The drawing under review shows one solid part. Ordinate dimensions are in mm from its lowest x, y, z. A direction names the side the tool comes from. Coordinates: 2 decimals unless noted, no trailing zeros. Order: outer loops, then holes, each group sorted by start corner. A loop starts at its lowest first (then second) coordinate and runs counter-clockwise, first axis right, second up. Notation, with made-up numbers: (-29, -24.75) - (19, -24.75) arc R7 ccw to (19, -17.75) - close; hole circle Ø4 at (67.5, -38). An arc over 180 degrees is marked (long way). Write item = value, one per line. Start each with the question number.
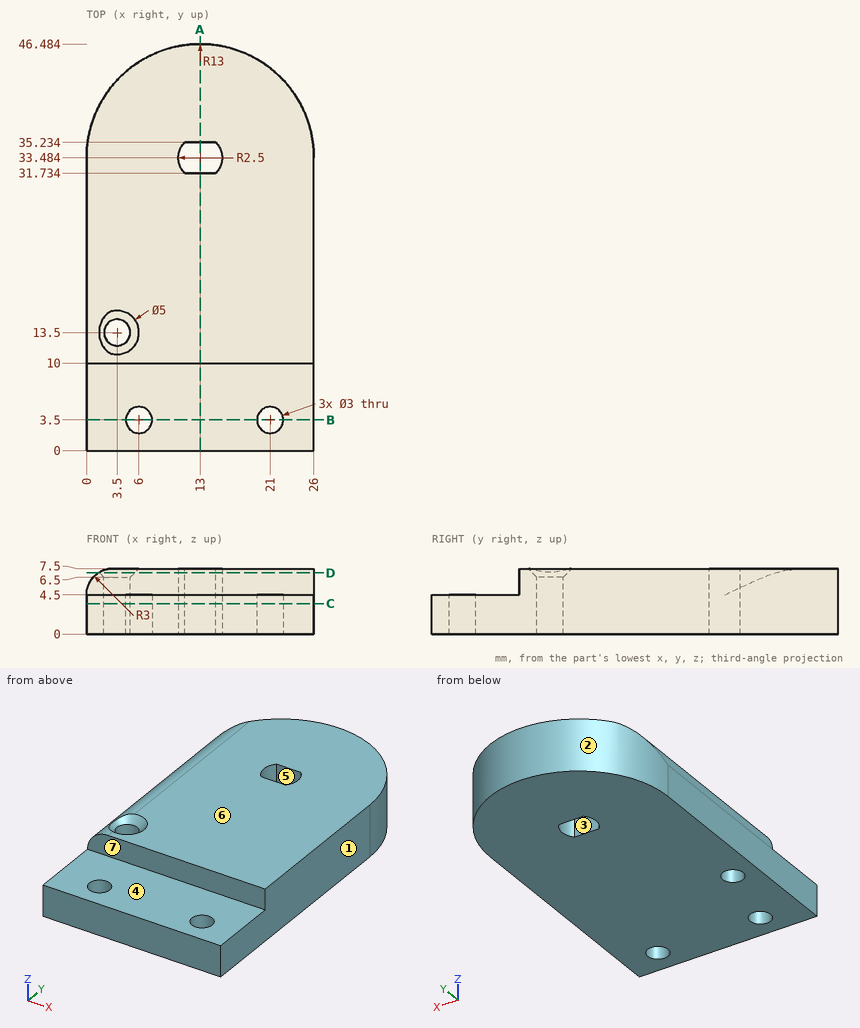
Item 1: For line 1 (X direction, y = 13.5, z = 4); line 2 (Y direction, x = 3.5, z = 2.25); line 3 (Y direction, x = 4, z = 5.75), list the stretches that pass through material, from the lowest coordinate up.
Item 2: For the marked faces 5, 6 and 7, list the 3-axis set-ups (+Z, -Z, +X, -X, +Y, -Y) from which the entire face can be reached by the end or side of a thin tool; tool diameter is ignored.
Item 3: Mouldability with a two-part tool opening along X and no side actions: class the marked faces 1, 2, 3 and 4 as +X half, -X half, draft (parallel to the pull), parting line (faces both ways), or undercut.
Item 4: For P1, Ø5, axis at x = 6, y = 3.5, coming from the +Z side; P2, Ø1.5, axis at x = 15.5, z = 6.5, coming from the -Y side; P3, Ø3, axis at y = 40.5, z = 4, coming from the -X side; P4, Ø1.8, axis at x = 21, y = 3.5, coming from the -Z side, all flat-tipped, find the tip position at first contact; note any pin that passes through.
Item 5: Add section A-A on x = 13. Give the boundary of the cut face in (y, z).
Item 6: Add section B-B on y = 3.5. Give the boundary of the cut face in (x, z), plus the area to 3 significant figures.
Item 7: Add section D-D on z = 7. Give the boundary of the cut face in (x, y), plus the area to 3 significant figures.
Item 8: Add section C-C on z = 3.5. Give the boundary of the cut face in (x, y), plus the area to 3 significant figures.
Worked out:
q1.line_1 = 0 to 2, 5 to 26
q1.line_2 = 0 to 12, 15 to 42.36
q1.line_3 = 10 to 12.09, 14.91 to 42.86
q2.face_5 = +Z, -Z
q2.face_6 = +Z, +X, -X, +Y, -Y
q2.face_7 = +Z, +X, -X, -Y
q3.face_1 = +X half
q3.face_2 = parting line
q3.face_3 = undercut
q3.face_4 = draft
q4.P1 = 4.5
q4.P2 = 10
q4.P3 = 1.23
q4.P4 = through
q5.outline = (0, 0) - (31.73, 0) - (31.73, 7.5) - (10, 7.5) - (10, 4.5) - (0, 4.5) - close; (35.23, 0) - (46.48, 0) - (46.48, 7.5) - (35.23, 7.5) - close
q6.outline = (0, 0) - (4.5, 0) - (4.5, 4.5) - (0, 4.5) - close; (7.5, 0) - (19.5, 0) - (19.5, 4.5) - (7.5, 4.5) - close; (22.5, 0) - (26, 0) - (26, 4.5) - (22.5, 4.5) - close
q6.area = 90.0 mm2
q7.outline = (1.34, 10) - (26, 10) - (26, 33.48) arc R13 ccw to (1.34, 39.24) - close; hole circle Ø4 at (3.5, 13.5); hole (11.21, 31.73) - (14.79, 31.73) arc R2.5 ccw to (14.79, 35.23) - (11.21, 35.23) arc R2.5 ccw to start
q7.area = 811 mm2
q8.outline = (0, 0) - (26, 0) - (26, 33.48) arc R13 ccw to (0, 33.48) - close; hole circle Ø3 at (3.5, 13.5); hole circle Ø3 at (6, 3.5); hole (11.21, 31.73) - (14.79, 31.73) arc R2.5 ccw to (14.79, 35.23) - (11.21, 35.23) arc R2.5 ccw to start; hole circle Ø3 at (21, 3.5)
q8.area = 1,100 mm2
